Autodesk Inventor part; units mm, degrees
ref_plane "YZ Plane" through (0, 0, 0) normal (1, 0, 0) x (0, 1, 0)
ref_plane "XZ Plane" through (0, 0, 0) normal (0, 1, 0) x (-1, 0, 0)
ref_plane "XY Plane" through (0, 0, 0) normal (0, 0, 1) x (1, 0, 0)
sketch "Эскиз1" plane through (0, 0, 0) normal (0, 0, 1) x (1, 0, 0)
  circle A0 centre (0, 0) radius 12.5
  dimension "d0" = 25
extrude "Выдавливание1" add sketch "Эскиз1" against normal blind 31
fillet "Сопряжение1" radius 1 1 edges at (-12.5, 0, 0)
sketch "Эскиз2" plane through (0, 0, 0) normal (0, 0, 1) x (1, 0, 0)
  circle A0 centre (0, 0) radius 12.5
  dimension "d4" = 25
extrude "Выдавливание2" add sketch "Эскиз2" along normal blind 25
sketch "Эскиз3" plane through (0, 0, 25) normal (0, 0, 1) x (1, 0, 0)
  circle A0 centre (0, 0) radius 3.5
  dimension "d7" = 7
extrude "Выдавливание3" add sketch "Эскиз3" along normal blind 2.5
sketch "Эскиз4" plane through (0, 0, 27.5) normal (0, 0, 1) x (1, 0, 0)
  circle A0 centre (0, 0) radius 2
  dimension "d10" = 4
extrude "Выдавливание4" add sketch "Эскиз4" along normal blind 1.5
sketch "Эскиз5" plane through (0, 0, 29) normal (0, 0, 1) x (1, 0, 0)
  arc A0 (1.3229, -1.5) -> (-1.3229, -1.5) centre (0, 0) ccw
  line L0 (0, 0) -> (0, 2)
  line L1 (1.3229, -1.5) -> (-1.3229, -1.5)
  circle A1 centre (0, 0) radius 2
  dimension "d14" = 3.5
extrude "Выдавливание5" add sketch "Эскиз5" along normal blind 8 contours L1 A0
sketch "Эскиз6" plane through (0, 0, 25) normal (0, 0, 1) x (1, 0, 0)
  circle A0 centre (0, 0) radius 8.5
  circle A1 centre (0, -8.5) radius 1.5
  dimension "d17" = 17
  dimension "d18" = 3
extrude "Выдавливание6" cut sketch "Эскиз6" against normal blind 5 contours A1 A0 | A0 A1 picked at (0, -7.9902) picked at (0.04, -8.9886)
pattern_circular "Круговой массив1" count 2 over 360 about axis through (0, 0, 0) along (0, 0, 1) of "Выдавливание6"
properties part number "Двигун"
Verification items for the finished model (mm, model axes). A direction names the side the tool comes from. Round coordinates to 2 decimals unless told otherwise and drop trailing zeros. Order: outer loops, then holes, each group sorted by start corner. A loop starts at its lowest first (then second) coordinate and runs counter-clockwise, first axis right, second up. Notation, with made-up numbers: (30, 58) - (65, 58) arc R36 cw to (65, 96) - close; hole circle Ø10 at (76, 57). An arc over 180 degrees is marked (long way). Use CSV: the item, a comma, the result in double quotes.
(1) Mould release check, pull along X, two halves, no side actions. Record for faces 1 (the face through (11.923, -3.755, 12.325)), 2 (the face through (0, -1.5, 33)), 3 (the face through (0, -10, 23)): released by +X, released by -X, zero draft, split by the parting line, or undercut.
Entries:
face 1,"split by the parting line"
face 2,"zero draft"
face 3,"undercut"
(2) Thickness scan on probe 1 along Y at (x, z) = (0, 22.55); probe 2 along Z at (x, y) = (-1, 5.5); probe 3 along Z at (x, y) = (-1.5, 1.75). Record the ranges inside material, lowest first. Write a range as from..to.
Entries:
probe 1,"-12.5..-10, -7..7, 10..12.5"
probe 2,"-31..25"
probe 3,"-31..27.5"
(3) Section check C-C on z = -16.5. Record the boundary of the cut face in (x, y).
Entries:
outline,"circle Ø25 at (0, 0)"
(4) Section check A-A on x = 0. Record the boundary of the cut face in (y, z), and give its area (3 significant figures).
Entries:
outline,"(-12.5, -31) - (12.5, -31) - (12.5, -1) arc R1 ccw to (11.5, 0) - (12.5, 0) - (12.5, 25) - (10, 25) - (10, 20) - (7, 20) - (7, 25) - (3.5, 25) - (3.5, 27.5) - (2, 27.5) - (2, 37) - (-1.5, 37) - (-1.5, 29) - (-2, 29) - (-2, 27.5) - (-3.5, 27.5) - (-3.5, 25) - (-7, 25) - (-7, 20) - (-10, 20) - (-10, 25) - (-12.5, 25) - (-12.5, 0) - (-11.5, 0) arc R1 ccw to (-12.5, -1) - close"
area,"1,420 mm^2"
(5) Section check D-D on z = 31.5. Record the boundary of the cut face in (x, y), and give its area (3 significant figures).
Entries:
outline,"(-1.32, -1.5) - (1.32, -1.5) arc R2 ccw (long way) to start"
area,"11.7 mm^2"
(6) Access from +Z, -Z, +X, -X, +Y, -Y to the whole of each face (thin tool, end or side, straight path). Record for faces 4 (the face through (3, -3, 25)), 5 (the face through (0, 0, -31)).
Entries:
face 4,"+Z"
face 5,"-Z, +X, -X, +Y, -Y"
(7) Gauge pin test, flat ends, axial feed: pin 1 Ø3 at (x, z) = (-5.5, 7) entering from +Y; pin 2 Ø1 at (y, z) = (4.5, -19) entering from +X; pin 3 Ø1.5 at (x, z) = (-3, 17) entering from +Y. Record the tip position at first contact, or that the pin passes through.
Entries:
pin 1,"y = 11.84"
pin 2,"x = 11.84"
pin 3,"y = 12.3"
(8) Section check B-B on y = 0. Record the boundary of the cut face in (x, z).
Entries:
outline,"(-12.5, -31) - (12.5, -31) - (12.5, -1) arc R1 ccw to (11.5, 0) - (12.5, 0) - (12.5, 25) - (3.5, 25) - (3.5, 27.5) - (2, 27.5) - (2, 37) - (-2, 37) - (-2, 27.5) - (-3.5, 27.5) - (-3.5, 25) - (-12.5, 25) - (-12.5, 0) - (-11.5, 0) arc R1 ccw to (-12.5, -1) - close"
